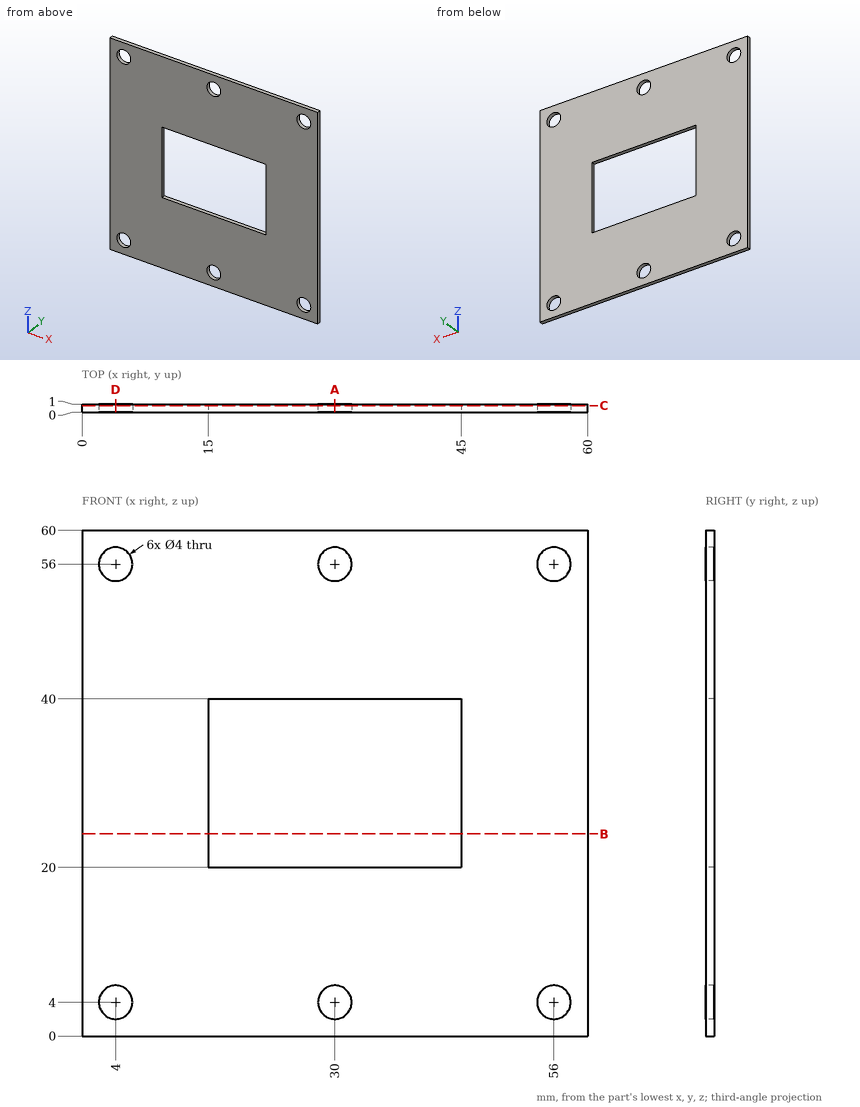
Answer from the drawing. Dimensions are ordinates in mm from the lowest x, y and z of the part. Give positions to 0.01 mm unless a question says otherwise; leave off trailing zeros. Order: outer loops, then holes, each group sorted by start corner. A loop starts at its lowest first (then second) coordinate and runs counter-clockwise, first axis right, second up. Notation, with made-up numbers: (48, -30) - (59, -30) arc R19 ccw to (59, -7) - close; hole circle Ø9 at (72, 22.25). An arc over 180 degrees is marked (long way). One line per item, written item: value. Start each with the question number.
1. Section D-D, the plane x = 4 is taken. Write down the section's boundary in (y, z).
2. Section C-C, the plane y = 0.8 is taken. Write down the section's boundary in (x, z), then the cut area to 3 significant figures.
3. Section B-B, the plane z = 24 is taken. Write down the section's boundary in (x, y).
4. Consider line 1 (X direction, y = 0.3, z = 4); line 2 (Z direction, x = 4, y = 0.35); line 3 (X direction, y = 0.95, z = 29). Determine where each line is inside the solid, lowest interval first.
5. Section A-A, the plane x = 30 is taken. Write down the section's boundary in (y, z), then the cut area to 3 significant figures.
Filled sheet:
1. outline: (0, 0) - (1, 0) - (1, 2) - (0, 2) - close; (0, 6) - (1, 6) - (1, 54) - (0, 54) - close; (0, 58) - (1, 58) - (1, 60) - (0, 60) - close
2. outline: (0, 0) - (60, 0) - (60, 60) - (0, 60) - close; hole circle Ø4 at (4, 4); hole circle Ø4 at (4, 56); hole (15, 20) - (45, 20) - (45, 40) - (15, 40) - close; hole circle Ø4 at (30, 4); hole circle Ø4 at (30, 56); hole circle Ø4 at (56, 4); hole circle Ø4 at (56, 56)
2. area: 2,920 mm²
3. outline: (0, 0) - (15, 0) - (15, 1) - (0, 1) - close; (45, 0) - (60, 0) - (60, 1) - (45, 1) - close
4. line 1: 0 to 2, 6 to 28, 32 to 54, 58 to 60
4. line 2: 0 to 2, 6 to 54, 58 to 60
4. line 3: 0 to 15, 45 to 60
5. outline: (0, 0) - (1, 0) - (1, 2) - (0, 2) - close; (0, 6) - (1, 6) - (1, 20) - (0, 20) - close; (0, 40) - (1, 40) - (1, 54) - (0, 54) - close; (0, 58) - (1, 58) - (1, 60) - (0, 60) - close
5. area: 32.0 mm²
